```python
from build123d import *

# Parameters (mm, degrees)
F0_W      = 112.7125
F0_H      = 76.2
F1_DEPTH  = 1.5875
F2_W      = 63.5
F2_H      = 38.1
F2_R      = 9.906
F3_DEPTH  = 1.5885
F4_W      = 112.7125
F4_H      = 1.5875
F5_DEPTH  = 63.5
F6_W      = 112.7125
F6_H      = 1.5875
F7_DEPTH  = 19.05
F8_R      = 2.54
F9_R      = 3.776515
F10_DEPTH = 1.5885


with BuildPart() as f1:
    # F0 (on Top) → F1 (new body)
    with BuildSketch(Plane.XY):
        with Locations((0.00635, 0)):
            Rectangle(F0_W, F0_H)
    extrude(amount=F1_DEPTH)

    # F2 (on face) → F3 (cut, through all)
    with BuildSketch(Plane.XY.offset(1.5875)):
        with Locations((-18.2499, 12.7)):
            Rectangle(F2_W, F2_H)
        with Locations((37.3126, 24.13)):
            Circle(F2_R)
        with Locations((37.3126, -0.127)):
            Circle(F2_R)
        with Locations((37.3126, -24.384)):
            Circle(F2_R)
        with Locations((-40.0939, -24.384)):
            Circle(F2_R)
        with Locations((-13.9319, -24.384)):
            Circle(F2_R)
        with Locations((12.2301, -24.384)):
            Circle(F2_R)
    extrude(amount=-F3_DEPTH, mode=Mode.SUBTRACT)

    # F4 (on face) → F5 (join)
    with BuildSketch(Plane.XY.offset(1.5875)):
        with Locations((0.00635, -38.89375)):
            Rectangle(F4_W, F4_H)
    extrude(amount=-F5_DEPTH)

    # F6 (on face) → F7 (join)
    with BuildSketch(Plane(origin=(0, -38.1, 0), x_dir=(-1, 0, 0), z_dir=(0, 1, 0))):
        with Locations((-0.00635, -61.11875)):
            Rectangle(F6_W, F6_H)
    extrude(amount=F7_DEPTH)

    # F8
    f8_edges = [f1.edges().sort_by_distance(p)[0] for p in [
        (0.00635, -39.6875, 1.5875),
        (0.00635, -38.1, 0),
        (0.00635, -39.6875, -61.9125),
        (0.00635, -38.1, -60.325),
    ]]
    fillet(f8_edges, radius=F8_R)

    # F9 (on face) → F10 (cut, through all)
    with BuildSketch(Plane.XY.offset(-60.325)):
        with Locations((-39.533325, -27.305)):
            Circle(F9_R)
        with Locations((-14.133325, -27.305)):
            Circle(F9_R)
        with Locations((11.266675, -27.305)):
            Circle(F9_R)
        with Locations((36.666675, -27.305)):
            Circle(F9_R)
    extrude(amount=-F10_DEPTH, mode=Mode.SUBTRACT)


solid = f1.part
```
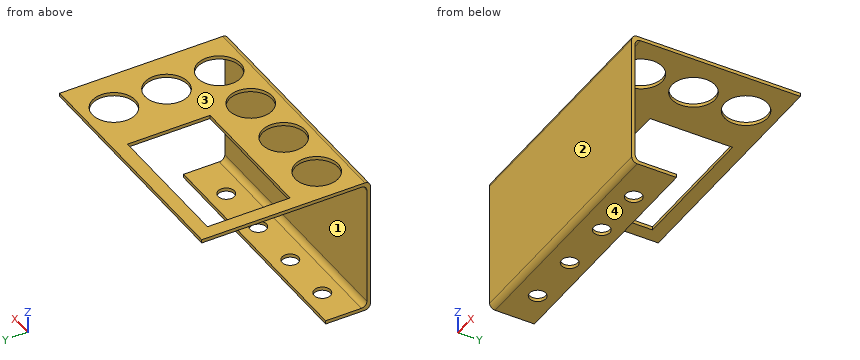
The listing builds one solid part. Answer for the finished solid, in the listing's coordinates (mm). Face numbers are marked on the shaded views. Coordinates: 2 decimals unless noted, no trailing zeros. Loops run counter-clockwise (first coordinate to the right, second up) from the corner with the lowest first, then second, coordinate; pieces in that order, holes last. Notation, with made-up numbers: M 55,-19.5 L 104,-19.5 A9 cw 104,-9.5 Z; hole C 29.25,65 d7. An arc over 180 degrees is marked long. Answer as a JSON object with one key per item and string values. Group by question number.
Item 1: Determine the mould class of the marked faces 1, 2, 3 and 4 for opening direction Z: +Z half, -Z half, draft (parallel to the pull), parting line (faces both ways), or undercut.
Item 2: Consider L1, parallel to Z at x = -28.5, y = -35 (1 decimal); L2, parallel to Y at x = 1, z = -19; L3, parallel to Z at x = 16, y = -24 (1 decimal). Determine where each line is inside the solid, lowest interval first.
Item 3: Each of these flat-tipped pins is pushed along its axis until it touches: P1, Ø12, axis at x = 37.31, y = -24.38, coming from the -Z side; P2, Ø2, axis at x = 0, z = -17, coming from the +Y side; P3, Ø13, axis at x = -11, y = -25.5, coming from the +Z side (3 decimals); P4, Ø1.3, axis at x = -20.5, z = -61, coming from the +Y side. Where does it stop, or does it pass through?
Item 4: Section D-D (x = 4) is taken. Give the number of separate pieces and of enclosed holes in the cut face, and give its area (3 significant figures).
Item 5: Section A-A (y = 24.13) is taken. Write down the section's boundary in (x, z), and give its area (3 significant figures).
Item 6: Section C-C (y = -20.5) is taken. Write down the section's boundary in (x, z) (1 decimal).
Solved:
{
 "1": {"face 1": "undercut", "face 2": "draft", "face 3": "+Z half", "face 4": "-Z half"},
 "2": {"L1": "z = -61.9 to -60.3, 0 to 1.6", "L2": "y = -39.69 to -38.1", "L3": "z = -61.9 to -60.3"},
 "3": {"P1": "stops at z = -61.91", "P2": "stops at y = -38.1", "P3": "stops at z = -60.325", "P4": "stops at y = -19.05"},
 "4": {"separate pieces": "3", "enclosed holes": "0", "area": "174 mm2"},
 "5": {"outline": "M -56.35,0 L -50,0 L -50,1.59 L -56.35,1.59 Z; M 13.5,0 L 27.41,0 L 27.41,1.59 L 13.5,1.59 Z; M 47.22,0 L 56.36,0 L 56.36,1.59 L 47.22,1.59 Z", "area": "46.7 mm2"},
 "6": {"outline": "M -56.3,-61.9 L 56.4,-61.9 L 56.4,-60.3 L -56.3,-60.3 Z; M -56.3,0 L -49.2,0 L -49.2,1.6 L -56.3,1.6 Z; M -31,0 L -23,0 L -23,1.6 L -31,1.6 Z; M -4.8,0 L 3.1,0 L 3.1,1.6 L -4.8,1.6 Z; M 21.3,0 L 28.2,0 L 28.2,1.6 L 21.3,1.6 Z; M 46.4,0 L 56.4,0 L 56.4,1.6 L 46.4,1.6 Z"}
}
